```python
from build123d import *

# Parameters (mm, degrees)
ESQUISSE1_R             = 11.2
ESQUISSE1_R_2           = 1.75
BOSS_EXTRU_1_DEPTH      = 10
BOSS_EXTRU_2_START      = -3
ESQUISSE2_R             = 11.2
ESQUISSE2_R_2           = 10.2
BOSS_EXTRU_2_DEPTH      = 3
ESQUISSE3_R             = 1.75
ENL_V_MAT_EXTRU_1_DEPTH = 44.588989435


with BuildPart() as part:
    # Esquisse1 → Boss.-Extru.1 (new body)
    with BuildSketch(Plane.XY):
        Polygon((-20, -10), (-20, 15), (20, 15), (20, -10), (30, -10), (30, -15), (-30, -15), (-30, -10), align=None)
        Circle(ESQUISSE1_R, mode=Mode.SUBTRACT)
        with Locations((15, 10)):
            Circle(ESQUISSE1_R_2, mode=Mode.SUBTRACT)
        with Locations((-15, 10)):
            Circle(ESQUISSE1_R_2, mode=Mode.SUBTRACT)
        with Locations((-15, -10)):
            Circle(ESQUISSE1_R_2, mode=Mode.SUBTRACT)
        with Locations((15, -10)):
            Circle(ESQUISSE1_R_2, mode=Mode.SUBTRACT)
    extrude(amount=BOSS_EXTRU_1_DEPTH)

    # Esquisse2 → Boss.-Extru.2 (add)
    with BuildSketch(Plane.XY.offset(10).offset(BOSS_EXTRU_2_START)):
        Circle(ESQUISSE2_R)
        Circle(ESQUISSE2_R_2, mode=Mode.SUBTRACT)
    extrude(amount=BOSS_EXTRU_2_DEPTH)

    # Esquisse3 → Enlèv. mat.-Extru.1 (cut, through all)
    with BuildSketch(Plane.XZ.offset(15)):
        with Locations(Location((-25, 5, 0), (0, 0, 270))):
            Circle(ESQUISSE3_R)
        with Locations((-15, 5)):
            Circle(ESQUISSE3_R)
        with Locations(Location((-5, 5, 0), (0, 0, 270))):
            Circle(ESQUISSE3_R)
        with Locations(Location((5, 5, 0), (0, 0, 270))):
            Circle(ESQUISSE3_R)
        with Locations((15, 5)):
            Circle(ESQUISSE3_R)
        with Locations(Location((25, 5, 0), (0, 0, 270))):
            Circle(ESQUISSE3_R)
    extrude(amount=-ENL_V_MAT_EXTRU_1_DEPTH, mode=Mode.SUBTRACT)


solid = part.part
```
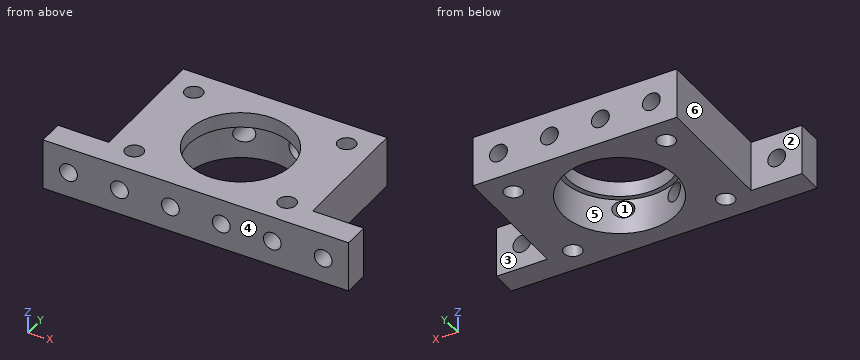
Can you work these out from the model? Positions are in its coordinate system, mm. Face numbers are marked on the shaded views. A direction names the side the tool comes from. Round coordinates to 2 decimals unless told otherwise and drop trailing zeros. Loops run counter-clockwise (first coordinate to the right, second up) from the corner with the lowest first, then second, coordinate; pieces in that order, holes last.
Item 1: Suppose I cut it at A-A, the plane y = 0. Write out the boundary of the cut face in (x, z).
Item 2: Which directions (+Z, -Z, +X, -X, +Y, -Y) give clear straight access to the entire face, cutting with the end or side of a thin tool? Please do the marked faces 1, 2 and 3.
Item 3: Suppose I cut it at B-B, the plane x = 0. Write out the boundary of the cut face in (y, z).
Item 4: Suppose I cut it at C-C, the plane z = 1.5. Write out the boundary of the cut face in (x, y).
Item 5: If we mould it in two halves opening along X, with no side actions, what happens to the marked faces 4, 5 and 6? For each: +X half, -X half, draft (parallel to the pull), parting line (faces both ways), or undercut.
Item 6: Suppose I cut it at D-D, the plane x = -15. Write out the boundary of the cut face in (y, z), then the cut area to 4 significant figures.
Item 7: Please list where these lines run through material, in increasing order: L1, parallel to Y at x = -15, z = 2.1; L2, parallel to Y at x = -16.5, z = 1.75; L3, parallel to Z at x = -15, y = 0.
Item 8: Will these pins go through, and if not, where does the flat tip stop? pin 1 Ø4 at (y, z) = (11, 5.5) entering from -X; pin 2 Ø3 at (x, z) = (26.5, 4) entering from +Y.
Reported:
1. outline: (-20, 0) - (-11.2, 0) - (-11.2, 7) - (-10.2, 7) - (-10.2, 10) - (-20, 10) - close; (10.2, 7) - (11.2, 7) - (11.2, 0) - (20, 0) - (20, 10) - (10.2, 10) - close; hole circle Ø3.5 at (-15, 5); hole circle Ø3.5 at (15, 5)
2. face 1: +Y, -Y
2. face 2: +Z, -Z, -X, +Y
2. face 3: +Z, -Z, +X, +Y
3. outline: (-15, 0) - (-11.2, 0) - (-11.2, 7) - (-10.2, 7) - (-10.2, 10) - (-15, 10) - close; (10.2, 7) - (11.2, 7) - (11.2, 0) - (15, 0) - (15, 10) - (10.2, 10) - close
4. outline: (-30, -15) - (30, -15) - (30, -10) - (20, -10) - (20, 15) - (-20, 15) - (-20, -10) - (-30, -10) - close; hole circle Ø3.5 at (-15, -10); hole circle Ø3.5 at (-15, 10); hole circle Ø22.4 at (0, 0); hole circle Ø3.5 at (15, -10); hole circle Ø3.5 at (15, 10)
5. face 4: draft
5. face 5: undercut
5. face 6: -X half
6. outline: (-15, 0) - (-11.75, 0) - (-11.75, 3.25) - (-15, 3.25) - close; (-15, 6.75) - (-11.75, 6.75) - (-11.75, 10) - (-15, 10) - close; (-8.25, 0) - (8.25, 0) - (8.25, 3.25) - (-8.25, 3.25) - close; (-8.25, 6.75) - (8.25, 6.75) - (8.25, 10) - (-8.25, 10) - close; (11.75, 0) - (15, 0) - (15, 3.25) - (11.75, 3.25) - close; (11.75, 6.75) - (15, 6.75) - (15, 10) - (11.75, 10) - close
6. area: 149.5 mm2
7. L1: y = -15 to -11.75, -8.25 to 8.25, 11.75 to 15
7. L2: y = -15 to -10.9, -9.1 to 9.1, 10.9 to 15
7. L3: z = 0 to 3.25, 6.75 to 10
8. pin 1: stops at x = -20
8. pin 2: stops at y = -10
